Design review of the part built by this model. Coordinates are the model's own, in mm. Face numbers are marked on the shaded views. A direction names the side the tool comes from. Coordinates: 2 decimals unless noted, no trailing zeros. Loops run counter-clockwise (first coordinate to the right, second up) from the corner with the lowest first, then second, coordinate; pieces in that order, holes last. Notation, with made-up numbers: M 52.25,39.5 L 63.25,39.5 A28 cw 63.25,63.5 Z; hole C 74.25,-29 d9. An arc over 180 degrees is marked long. One line per item, written item: value.
```python
from build123d import *

# Parameters (mm, degrees)
BASE_FLANGE1_DEPTH       = 1
SKETCHED_START           = 21.616422755
SKETCHED_BEND1_OUTLINE_W = 40
SKETCHED_BEND1_OUTLINE_H = 1
SKETCHED_BEND1_DEPTH     = 28.383577245
SKETCHED_START_2         = 20.821902755
SKETCHED_BEND1_2_DEPTH   = 0.00548
SKETCHED_START_3         = 19.821902755
SKETCHED_BEND1_3_DEPTH   = 2
SKETCHED_START_4         = -20
SKETCHED_BEND1_4_DEPTH   = 40
SKETCH7_R                = 3.025
CUT_EXTRUDE1_DEPTH       = 10
F_6_CLEARANCE_HOLE1_D    = 3.7973
F_4_CLEARANCE_HOLE2_D    = 3.2639


with BuildPart() as part:
    # Base-Flange1: sheet metal written as solids
    # Sketch1 → Base-Flange1 (new body)
    with BuildSketch(Plane(origin=(0, 0, 0), x_dir=(1, 0, 0), z_dir=(0, 1, 0))):
        with BuildLine():
            Line((-20, -18), (-20, -45))
            ThreePointArc((-20, -45), (-18.535533906, -48.535533906), (-15, -50))
            Line((-15, -50), (15, -50))
            ThreePointArc((15, -50), (18.535533906, -48.535533906), (20, -45))
            Line((20, -45), (20, -18))
            Line((20, -18), (26, -18))
            ThreePointArc((26, -18), (27.414213562, -17.414213562), (28, -16))
            Line((28, -16), (28, -4))
            ThreePointArc((28, -4), (27.414213562, -2.585786438), (26, -2))
            Line((26, -2), (20, -2))
            Line((20, -2), (20, 35))
            ThreePointArc((20, 35), (15.606601718, 45.606601718), (5, 50))
            Line((5, 50), (-5, 50))
            ThreePointArc((-5, 50), (-15.606601718, 45.606601718), (-20, 35))
            Line((-20, 35), (-20, -2))
            Line((-20, -2), (-26, -2))
            ThreePointArc((-26, -2), (-27.414213562, -2.585786438), (-28, -4))
            Line((-28, -4), (-28, -16))
            ThreePointArc((-28, -16), (-27.414213562, -17.414213562), (-26, -18))
            Line((-26, -18), (-20, -18))
        make_face()
    extrude(amount=-BASE_FLANGE1_DEPTH)

    # Sketched Bend1: read off the stored shape, not the designer's step
    # Sketched Bend1 outline → Sketched Bend1 (cut)
    with BuildSketch(Plane.XY.offset(SKETCHED_START)):
        with Locations((0, -0.5)):
            Rectangle(SKETCHED_BEND1_OUTLINE_W, SKETCHED_BEND1_OUTLINE_H)
    extrude(amount=SKETCHED_BEND1_DEPTH, mode=Mode.SUBTRACT)

    # Sketched Bend1 2 outline → Sketched Bend1 2 (add)
    with BuildSketch(Plane.XY.offset(SKETCHED_START_2)):
        with BuildLine():
            Line((20, 0), (20, 23.821902755))
            ThreePointArc((20, 23.821902755), (18.535533906, 27.357436661), (15, 28.821902755))
            Line((15, 28.821902755), (-15, 28.821902755))
            ThreePointArc((-15, 28.821902755), (-18.535533906, 27.357436661), (-20, 23.821902755))
            Line((-20, 23.821902755), (-20, 0))
            Line((-20, 0), (20, 0))
        make_face()
    extrude(amount=SKETCHED_BEND1_2_DEPTH)

    # Sketched Bend1 3 outline → Sketched Bend1 3 (add)
    with BuildSketch(Plane.XY.offset(SKETCHED_START_3)):
        with BuildLine():
            Line((20, 0), (20, 23.821902755))
            ThreePointArc((20, 23.821902755), (18.535533906, 27.357436661), (15, 28.821902755))
            Line((15, 28.821902755), (-15, 28.821902755))
            ThreePointArc((-15, 28.821902755), (-18.535533906, 27.357436661), (-20, 23.821902755))
            Line((-20, 23.821902755), (-20, 0))
            Line((-20, 0), (20, 0))
        make_face()
    extrude(amount=SKETCHED_BEND1_3_DEPTH)

    # Sketched Bend1 4 outline → Sketched Bend1 4 (cut)
    with BuildSketch(Plane.YZ.offset(SKETCHED_START_4)):
        with BuildLine():
            Line((28.821902755, 19.821902755), (28.821902755, 20.821902755))
            Line((28.821902755, 20.821902755), (1, 20.821902755))
            ThreePointArc((1, 20.821902755), (0.292893219, 20.529009536), (0, 19.821902755))
            Line((0, 19.821902755), (28.821902755, 19.821902755))
        make_face()
        with BuildLine():
            ThreePointArc((-1, 19.821902755), (-0.414213562, 21.236116317), (1, 21.821902755))
            Line((1, 21.821902755), (0, 21.821902755))
            Line((0, 21.821902755), (0, 21.616422755))
            Line((0, 21.616422755), (-1, 21.616422755))
            Line((-1, 21.616422755), (-1, 19.821902755))
        make_face()
    extrude(amount=SKETCHED_BEND1_4_DEPTH, mode=Mode.SUBTRACT)

    # Sketch7 → Cut-Extrude1 (cut)
    with BuildSketch(Plane(origin=(0, 0, 0), x_dir=(1, 0, 0), z_dir=(0, 1, 0))):
        with Locations(Location((0, -6.821902755, 0), (0, 0, 270))):
            Circle(SKETCH7_R)
        with Locations(Location((0, 35.578097245, 0), (0, 0, 270))):
            Circle(SKETCH7_R)
    extrude(amount=-CUT_EXTRUDE1_DEPTH, mode=Mode.SUBTRACT)

    # #6 Clearance Hole1 (through all)
    with Locations(Plane(origin=(0, 0, 20.821902755), x_dir=(-1, 0, 0), z_dir=(0, 0, -1))):
        with Locations((13, 6.681902755), (-13, 6.681902755), (0, 21.821902755)):
            Hole(F_6_CLEARANCE_HOLE1_D / 2)

    # #4 Clearance Hole2 (through all)
    with Locations(Plane(origin=(0, 0, 0), x_dir=(1, 0, 0), z_dir=(0, 1, 0))):
        with Locations((-24, -6), (-24, -14), (24, -6), (24, -14)):
            Hole(F_4_CLEARANCE_HOLE2_D / 2)


solid = part.part
```
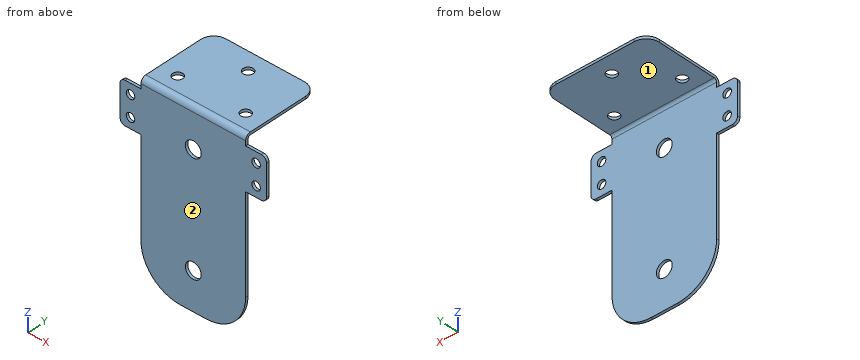
(1) We need section A-A on x = 0. State the section outline as (y, z) points, then the cut area to 3 significant figures.
Reply:
outline: M -1,-50 L 0,-50 L 0,-38.6 L -1,-38.6 Z; M -1,-32.55 L 0,-32.55 L 0,3.8 L -1,3.8 Z; M -1,9.85 L 0,9.85 L 0,19.82 A1 cw 1,20.82 L 19.92,20.82 L 19.92,21.82 L 1,21.82 A2 ccw -1,19.82 Z; M 23.72,20.82 L 28.82,20.82 L 28.82,21.82 L 23.72,21.82 Z
area: 84.1 mm2
(2) To check wall thickness, follow line 1 along X through (y, z) = (-0.45, 14); line 2 along X through (y, z) = (-0.15, 6); line 3 along Z through (x, y) = (12.5, 27.25). State the ranges of each line that lie inside material, in increasing order. Write a range as [from, to].
Reply:
line 1: x = [-28, -25.63], [-22.37, 22.37], [25.63, 28]
line 2: x = [-28, -25.63], [-22.37, -2.91], [2.91, 22.37], [25.63, 28]
line 3: z = [20.82, 21.82]
(3) We need section B-B on z = 14. State the section outline as (x, y) points.
Reply:
outline: M -28,-1 L -25.63,-1 L -25.63,0 L -28,0 Z; M -22.37,-1 L 22.37,-1 L 22.37,0 L -22.37,0 Z; M 25.63,-1 L 28,-1 L 28,0 L 25.63,0 Z
(4) Tool access review of the marked faces 1 and 2: name each direction out of +Z, -Z, +X, -X, +Y, -Y from which nothing blocks a thin tool from reaching the whole face with its end or side.
Reply:
face 1: -Z, +X, -X, +Y
face 2: +Z, -Z, +X, -X, -Y
(5) We need section C-C on x = 24. State the section outline as (y, z) points.
Reply:
outline: M -1,2 L 0,2 L 0,4.37 L -1,4.37 Z; M -1,7.63 L 0,7.63 L 0,12.37 L -1,12.37 Z; M -1,15.63 L 0,15.63 L 0,18 L -1,18 Z
(6) Insertion check: pin 1 (0.8 mm diameter, centred on y = -0.5, z = -20.5, fed in from -X); pin 2 (3 mm diameter, centred on x = 5, y = 12.5, fed in from -Z); pin 3 (1.1 mm diameter, centred on y = -0.5, z = -23.5, fed in from +X); pin 4 (4 mm diameter, centred on x = -24, z = 6, fed in from -Y). Each pin has a flat end and moves straight along its axis. Give the tip position at first contact, or say it passes through.
Reply:
pin 1: stops at x = -20
pin 2: stops at z = 20.82
pin 3: stops at x = 20
pin 4: stops at y = -1
(7) We need section D-D on z = 6. State the section outline as (x, y) points.
Reply:
outline: M -28,-1 L -25.63,-1 L -25.63,0 L -28,0 Z; M -22.37,-1 L -2.91,-1 L -2.91,0 L -22.37,0 Z; M 2.91,-1 L 22.37,-1 L 22.37,0 L 2.91,0 Z; M 25.63,-1 L 28,-1 L 28,0 L 25.63,0 Z
